Autodesk Inventor part; units mm, degrees
ref_plane "YZ Plane" through (0, 0, 0) normal (1, 0, 0) x (0, 1, 0)
ref_plane "XZ Plane" through (0, 0, 0) normal (0, 1, 0) x (-1, 0, 0)
ref_plane "XY Plane" through (0, 0, 0) normal (0, 0, 1) x (1, 0, 0)
sketch "Sketch1" plane through (0, 0, 0) normal (0, 0, 1) x (1, 0, 0)
  line L0 (-12.1708, 16.0073) -> (13.2292, 16.0073)
  line L1 (13.2292, 16.0073) -> (13.2292, -34.7927)
  line L2 (13.2292, -34.7927) -> (-12.1708, -34.7927)
  line L3 (-12.1708, -34.7927) -> (-12.1708, 16.0073)
  line L4 (11.9592, 14.7373) -> (-10.9008, 14.7373)
  line L5 (-10.9008, 14.7373) -> (-10.9008, -33.5227)
  line L6 (-10.9008, -33.5227) -> (11.9592, -33.5227)
  line L7 (11.9592, -33.5227) -> (11.9592, 14.7373)
  point P0 (0, 0)
  dimension "d0" = 25.4
  dimension "d1" = 50.8
  dimension "d2" = 1.27
extrude "Extrusion1" add sketch "Sketch1" along normal blind 152.4
sketch "Sketch2" plane through (-12.1708, 16.0073, 0) normal (0, 1, 0) x (1, 0, 0)
  circle A0 centre (12.7, -12.7) radius 1.7272
  line L0 (25.4, 0) -> (0, 0)
  line L1 (0, 0) -> (0, -152.4)
  point P0 (12.1708, 0)
  dimension "d5" = 3.4544
  dimension "d6" = 12.7
  dimension "d7" = 12.7
extrude "Extrusion2" cut sketch "Sketch2" against normal through all
pattern_linear "Rectangular Pattern1" count 15 spacing 25.4 along (0, 0, 1) of "Extrusion2"
sketch "Sketch3" plane through (-12.1708, 16.0073, 0) normal (0, 1, 0) x (1, 0, 0)
  circle A0 centre (6.35, -6.35) radius 2.3813
  line L0 (25.4, 0) -> (0, 0)
  line L1 (0, 0) -> (0, -152.4)
  circle A1 centre (6.35, -146.05) radius 2.3813
  line L2 (25.4, -152.4) -> (0, -152.4)
  circle A2 centre (6.35, -120.65) radius 2.3813
  circle A3 centre (6.35, -31.75) radius 2.3813
  point P0 (12.1708, 0)
  dimension "d15" = 6.35
  dimension "d16" = 6.35
  dimension "d17" = 4.7625
  dimension "d18" = 6.35
  dimension "d19" = 6.35
  dimension "d20" = 4.7625
  dimension "d23" = 6.35
  dimension "d24" = 6.35
  dimension "d25" = 25.4
  dimension "d26" = 4.7625
  dimension "d27" = 25.4
  dimension "d28" = 4.7625
extrude "Extrusion3" cut sketch "Sketch3" against normal through all
sketch "Sketch4" plane through (13.2292, -34.7927, 0) normal (1, 0, 0) x (0, 0, -1)
  circle A0 centre (-76.2, 25.4) radius 9.525
  line L0 (0, 0) -> (-152.4, 0)
  line L1 (0, 0) -> (0, 50.8)
  point P0 (0, 34.7927)
  point P1 (0, 25.4)
  dimension "d29" = 25.4
  dimension "d30" = 76.2
  dimension "d31" = 19.05
extrude "Extrusion4" cut sketch "Sketch4" against normal through all
equation "\"d3\" = d13"
equation "\"d10\" = d14"
equation "\"d13\" = 152.4"
equation "\"d14\" = d13"
properties part number "VersaFrame (arm base)"
Source: CAD feature listing. Evaluate the final solid. Frame: model axes, mm. A direction names the side the tool comes from. Coordinates: 2 decimals unless noted, no trailing zeros. Loops run counter-clockwise (first coordinate to the right, second up) from the corner with the lowest first, then second, coordinate; pieces in that order, holes last. Notation, with made-up numbers: (62, 5) -> (107, 5) arc R18 ccw to (107, 38) -> close; hole circle Ø7 at (-28, 23). An arc over 180 degrees is marked (long way). Answer in a Markdown table with one row per item. Add a question column.
Q1. Ray query, line 1 along Y through (x, z) = (1, 121.5); line 2 along X through (y, z) = (-19, 15); line 3 along Y through (x, z) = (-11.15, 76.2). Return the intervals inside material, ascending.
Q2. Reachability of faces 1 (the face through (1, -34.793, 75)), 2 (the face through (11.959, 1, 75)) from +Z, -Z, +X, -X, +Y, -Y: full face, straight path, thin tool, end or side. Return the list, or none.
Q3. Section D-D on z = 110. Return the cut outline in (x, y), and give its area (3 significant figures).
Q4. Pull-direction query (X, two-part tool) for faces 3 (the face through (12.603, -8.974, 85.716)), 4 (the face through (13.229, -20, 75)), 5 (the face through (-10.901, -20, 75)); classes: pulls with the +X half, pulls with the -X half, needs draft (parallel to the pull), parting line crosses it, or undercut.
Q5. Section C-C on z = 146.05. Return the cut outline in (x, y).
Q6. Section B-B on y = -22.5. Return the cut outline in (x, z), and give its area (3 significant figures).
Q7. Section A-A on x = 5.25. Return the cut outline in (y, z).
Q8. Contact query for a flat-ended pin moving along its axis: pin 1 Ø3 at (x, z) = (0.53, 12.7) entering from -Y. Output: stop coordinate, or through.
Computed values:
| question | item | result |
|---|---|---|
| 1 | line 1 | y = -34.79 to -33.52, 14.74 to 16.01 |
| 1 | line 2 | x = -12.17 to -10.9, 11.96 to 13.23 |
| 1 | line 3 | y = -34.79 to -18.92, 0.13 to 16.01 |
| 2 | face 1 | +Z, -Z, +X, -X, -Y |
| 2 | face 2 | +Z, -Z |
| 3 | outline | (-12.17, -34.79) -> (13.23, -34.79) -> (13.23, 16.01) -> (-12.17, 16.01) -> close; hole (-10.9, -33.52) -> (11.96, -33.52) -> (11.96, 14.74) -> (-10.9, 14.74) -> close |
| 3 | area | 187 mm^2 |
| 4 | face 3 | needs draft |
| 4 | face 4 | pulls with the +X half |
| 4 | face 5 | undercut |
| 5 | outline | (-12.17, -34.79) -> (-8.2, -34.79) -> (-8.2, -33.52) -> (-10.9, -33.52) -> (-10.9, 14.74) -> (-8.2, 14.74) -> (-8.2, 16.01) -> (-12.17, 16.01) -> close; (-3.44, -34.79) -> (13.23, -34.79) -> (13.23, 16.01) -> (-3.44, 16.01) -> (-3.44, 14.74) -> (11.96, 14.74) -> (11.96, -33.52) -> (-3.44, -33.52) -> close |
| 6 | outline | (-12.17, 0) -> (-10.9, 0) -> (-10.9, 152.4) -> (-12.17, 152.4) -> close; (11.96, 0) -> (13.23, 0) -> (13.23, 152.4) -> (11.96, 152.4) -> close |
| 6 | area | 387 mm^2 |
| 7 | outline | (-34.79, 0) -> (-33.52, 0) -> (-33.52, 152.4) -> (-34.79, 152.4) -> close; (14.74, 0) -> (16.01, 0) -> (16.01, 152.4) -> (14.74, 152.4) -> close |
| 8 | pin 1 | passes through |
